Can you work these out from the model? Positions are in its coordinate system, mm. Face numbers are marked on the shaded views. A direction names the side the tool comes from. Give positions to 0.01 mm unless a question says otherwise; leave off trailing zeros. Order: outer loops, then holes, each group sorted by start corner. A loop starts at its lowest first (then second) coordinate and runs counter-clockwise, first axis right, second up. Notation, with made-up numbers: M 11.5,42 L 54.5,42 A27 ccw 54.5,63 Z; hole C -28.5,13 d3. An arc over 180 degrees is marked long. Write each question's results on one line, items separated by ' | '.
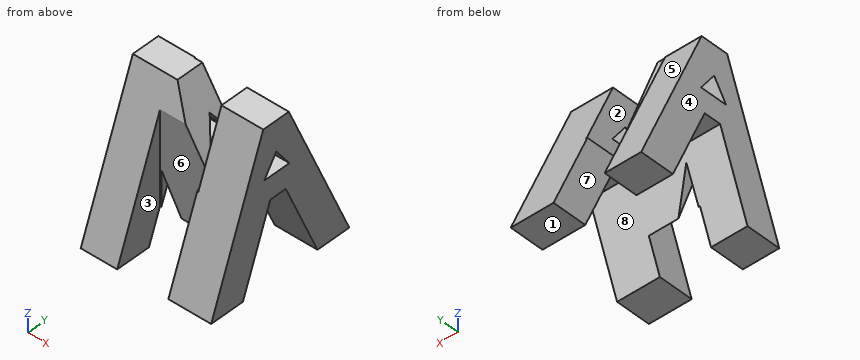
from build123d import *

# Parameters (mm, degrees)
F0_W     = 38.1
F0_H     = 38.1
F1_DEPTH = 38.1
F3_DEPTH = 38.1
F4_W     = 3.3369022369
F4_H     = 38.1
F4_W_2   = 1.9459760515
F5_DEPTH = 38.1
F6_W     = 1.9311041106
F6_H     = 38.1
F6_W_2   = 12.8730144352
F6_H_2   = 16.8606620282
F6_H_3   = 11.8112149596
F6_W_3   = 3.1704599917
F7_DEPTH = 38.1


with BuildPart() as f1:
    # F0 (on Front) → F1 (new body)
    with BuildSketch(Plane.XZ):
        with Locations((19.05, 19.05)):
            Rectangle(F0_W, F0_H)
    extrude(amount=F1_DEPTH)

    # F2 (on Right) → F3 (cut)
    with BuildSketch(Plane.YZ):
        Polygon((-38.1, 0), (-23.7257722765, 38.1), (-38.1, 38.1), align=None)
        Polygon((-29.3381027877, 0), (-8.7619078, 0), (-17.5237406998, 20.0202792485), (-21.7849255435, 20.0202792485), align=None)
        Polygon((-16.6743844748, 38.1), (0, 0), (0, 38.1), align=None)
        Polygon((-23.437961936, 25.6237238646), (-20.1281253248, 25.6237238646), (-16.5304783732, 25.6237238646), (-20.1281253248, 30.6604318321), align=None)
    extrude(amount=F3_DEPTH, mode=Mode.SUBTRACT)

    # F4 (on Front) → F5 (cut)
    with BuildSketch(Plane.XZ):
        with Locations((36.4315488815, 19.05)):
            Rectangle(F4_W, F4_H)
        Polygon((24.2471154779, 38.1), (13.187199831, 38.1), (24.2471154779, 20.9880266339), align=None)
        Polygon((11.5554118529, 16.8178956956), (11.3741010427, 0), (21.1648438126, 0), align=None)
        with Locations((0.9729880258, 19.05)):
            Rectangle(F4_W_2, F4_H)
    extrude(amount=F5_DEPTH, mode=Mode.SUBTRACT)

    # F6 (on Top) → F7 (cut)
    with BuildSketch(Plane.XY):
        with Locations((0.9655520553, -19.05)):
            Rectangle(F6_W, F6_H)
        with Locations((17.5597285852, -8.4303310141)):
            Rectangle(F6_W_2, F6_H_2)
        with Locations((17.5597285852, -32.1943925202)):
            Rectangle(F6_W_2, F6_H_3)
        with Locations((36.5147700042, -19.05)):
            Rectangle(F6_W_3, F6_H)
    extrude(amount=F7_DEPTH, mode=Mode.SUBTRACT)


solid = f1.part
(1) We'd pull the mould along X, two halves only. Please class the marked faces 1, 2, 3 and 4: +X half, -X half, draft (parallel to the pull), parting line (faces both ways), or undercut.
Data:
face 1: draft | face 2: undercut | face 3: undercut | face 4: -X half
(2) Imagine slicing it at D-D, the plane x = 19. Write out the boundary of the cut face in (y, z), plus the area to 3 significant figures.
Data:
outline: M -26.29,8.08 L -21.78,20.02 L -17.52,20.02 L -16.86,18.51 L -16.86,25.62 L -23.44,25.62 L -21.15,29.11 L -26.29,29.11 Z; M -19.02,29.11 L -16.86,26.09 L -16.86,29.11 Z | area: 97.4 mm2
(3) Imagine slicing it at B-B, the plane y = -2.5. Write out the boundary of the cut face in (x, z).
Data:
outline: M 1.95,0 L 11.12,0 L 11.12,5.71 L 1.95,5.71 Z; M 24,0 L 34.76,0 L 34.76,5.71 L 24,5.71 Z
(4) For the marked faces 5, 6, 7 and 8, which set-ups out of +Z, -Z, +X, -X, +Y, -Y let a thin tool reach every point of the face, with its end or its side?
Data:
face 5: +Z, +X, -X, +Y | face 6: +Z, -Z, -Y | face 7: +Z, -Z, +Y | face 8: -Z, +X, -X
(5) Imagine slicing it at C-C, the plane z = 22. Write out the boundary of the cut face in (x, y).
Data:
outline: M 1.95,-29.8 L 11.12,-29.8 L 11.12,-26.29 L 23.59,-26.29 L 23.59,-16.86 L 11.12,-16.86 L 11.12,-9.63 L 1.95,-9.63 Z; M 24.25,-29.8 L 34.76,-29.8 L 34.76,-9.63 L 24.25,-9.63 Z
(6) Will these pins go through, and if not, where does the flat tip stop? P1, Ø1.5, axis at x = 15, y = -21.5, coming from the +Z side; P2, Ø6.5, axis at x = 15.5, z = 17.5, coming from the -Y side; P3, Ø3.5, axis at x = 14, y = -19.5, coming from the -Z side; P4, Ø1, axis at x = 12.5, z = 5, coming from the -Y side.
Data:
P1: stops at z = 36.46 | P2: stops at y = -26.29 | P3: stops at z = 20.02 | P4: passes through
(7) I need wall thicknesses on L1, parallel to X at y = -6, z = 4; L2, parallel to Y at x = 25.5, z = 29; L3, parallel to Y at x = 26.5, z = 26.5. Which ranges of each line are inside material? Lowest first, please. Write a range as from..to.
Data:
L1: x = 1.95..11.12, 24..34.76 | L2: y = -27.16..-21.22, -18.94..-12.69 | L3: y = -28.1..-22.86, -17.16..-11.6
(8) Imagine slicing it at A-A, the plane x = 25.5. Write out the boundary of the cut face in (y, z), plus the area to 3 significant figures.
Data:
outline: M -38.1,0 L -29.34,0 L -21.78,20.02 L -17.52,20.02 L -8.76,0 L 0,0 L -16.67,38.1 L -23.73,38.1 Z; hole M -23.44,25.62 L -16.53,25.62 L -20.13,30.66 Z | area: 594 mm2
